The listing builds one solid part. Answer for the finished solid, in the listing's coordinates (mm). A direction names the side the tool comes from. Round coordinates to 2 decimals unless told otherwise and drop trailing zeros. Order: outer loops, then holes, each group sorted by start corner. A loop starts at its lowest first (then second) coordinate and runs counter-clockwise, first axis right, second up. Notation, with made-up numbers: M 84.25,57.25 L 111.25,57.25 A18 ccw 111.25,76.25 Z; hole C 3,19.25 d3. An arc over 180 degrees is marked long. Write item = value, one per line. Start each with the question number.
(1) A cutting plane is placed at B-B, the plane z = 83. Determine the outline of the cut face in (x, y), and give its area (3 significant figures).
(2) Which of the six approach directions +Z, -Z, +X, -X, +Y, -Y give full straight-line access (tool end or side, diameter ignored) to faces 1 (the face through (0, -17, 72.215)), 2 (the face through (0, 0, 5)), 3 (the face through (0, -3, 25)), 4 (the face through (-0.434, -36.93, 68.934))?
(3) A cutting plane is placed at D-D, the plane z = 98. Determine the outline of the cut face in (x, y) (1 decimal).
(4) A cutting plane is placed at A-A, the plane x = 5.75. Determine the outline of the cut face in (y, z), and give its area (3 significant figures).
(5) Straight lines are drawn through the part: probe 1 along Z at (x, y) = (-2.5, -22); probe 2 along Y at (x, z) = (-0.75, 79.5); probe 3 along Z at (x, y) = (-0.25, -35). For each, find the intervals that lie inside material, in ascending order. Write a range as from..to.
(6) A cutting plane is placed at C-C, the plane y = -16.5. Determine the outline of the cut face in (x, z).
(7) Each of these flat-tipped pins is pushed along its axis until it touches: pin 1 (12.5 mm diameter, centred on x = 1.5, z = 61, fed in from +Y); pin 2 (3 mm diameter, centred on x = 3.5, z = 69, fed in from -Y); pin 3 (6 mm diameter, centred on x = 8.5, y = -30.5, fed in from -Z). Where does it stop, or does it pass through?
Autodesk Inventor part; units mm, degrees
ref_plane "YZ Plane" through (0, 0, 0) normal (1, 0, 0) x (0, 1, 0)
ref_plane "XZ Plane" through (0, 0, 0) normal (0, 1, 0) x (-1, 0, 0)
ref_plane "XY Plane" through (0, 0, 0) normal (0, 0, 1) x (1, 0, 0)
sketch "Sketch1" plane through (0, 0, 0) normal (0, 0, 1) x (1, 0, 0)
  circle A0 centre (0, 0) radius 3
  dimension "d0" = 6
extrude "Extrusion1" add sketch "Sketch1" along normal blind 50
sketch "Sketch2" plane through (0, 0, 0) normal (0, 1, 0) x (-1, 0, 0)
  line L0 (-12.5, 75) -> (-12.5, 50)
  line L1 (-12.5, 50) -> (12.5, 50)
  line L2 (12.5, 50) -> (12.5, 75)
  line L3 (12.5, 75) -> (-12.5, 75)
  line L4 (-12.5, 75) -> (12.5, 50) construction
  line L5 (-12.5, 50) -> (12.5, 75) construction
  line L6 (3, 50) -> (-3, 50)
  line L7 (3, 50) -> (-3, 50)
  line L8 (3, 0) -> (-3, 0)
  line L9 (3, 0) -> (-3, 0)
  line L10 (-3, 0) -> (3, 50)
  line L11 (3, 0) -> (-3, 50)
  line L12 (12.5, 75) -> (3, 84.5)
  line L13 (3, 84.5) -> (3, 84.5)
  line L14 (3, 84.5) -> (-3, 84.5)
  line L15 (-3, 84.5) -> (-3, 84.5)
  line L16 (-3, 84.5) -> (-12.5, 75)
  line L17 (0.25, 84.5) -> (0, 114.5)
  line L18 (0, 114.5) -> (-0.25, 84.5)
  line L19 (0, 114.5) -> (0, 84.5)
  point P0 (0, 0)
  point P1 (0, 62.5)
  point P2 (0, 50)
  point P3 (0, 25)
  point P4 (0, 62.5)
  dimension "d3" = 25
  dimension "d4" = 25
  dimension "d5" = 6
  dimension "d6" = 0
  dimension "d11" = 30
  dimension "d14" = 0.5
  dimension "d15" = 0.25
extrude "Extrusion2" add sketch "Sketch2" along normal mid plane 4 contours L3 L2 L1 L0 | L16 L14 L12 L3
sketch "Sketch3" plane through (0, -2, 0) normal (0, -1, 0) x (1, 0, 0)
  line L0 (-10, 72.2148) -> (-10, 62.2148)
  line L1 (-10, 62.2148) -> (10, 62.2148)
  line L2 (10, 62.2148) -> (10, 72.2148)
  line L3 (10, 72.2148) -> (-10, 72.2148)
  line L4 (-10, 72.2148) -> (10, 62.2148) construction
  line L5 (-10, 62.2148) -> (10, 72.2148) construction
  point P0 (0, 0)
  point P1 (0, 67.2148)
  dimension "d18" = 10
  dimension "d24" = 20
extrude "Extrusion3" add sketch "Sketch3" along normal blind 30
revolve "Revolution1" add sketch "Sketch2" angle 360 about axis through (0, 0, 114.5) along (0, 0, -1) contours L14 L19 L17
sketch "Sketch5" plane through (0, 0, 0) normal (0, 0, -1) x (-1, 0, 0)
  arc A0 (-2.2361, 2) -> (-2.2361, -2) centre (0, 0) ccw
  line L0 (-3, 0) -> (3.9396, 0)
  line L1 (3.9396, 0) -> (3.9396, 5.4672)
  line L2 (3.9396, 5.4672) -> (-3, 5.4672)
  line L3 (-3, 5.4672) -> (-3, 0)
extrude "Extrusion4" cut sketch "Sketch5" against normal blind 10
sketch "Sketch6" plane through (0, -32, 0) normal (0, -1, 0) x (1, 0, 0)
  circle A0 centre (0, 66.9819) radius 2
  point P0 (0, 0)
  dimension "d25" = 4
extrude "Extrusion5" add sketch "Sketch6" along normal blind 10
equation "\"d15\" = 0.5 * d14"
properties part number "electrode"
Reported:
q1.outline = M -4.5,-2 L 4.5,-2 L 4.5,2 L -4.5,2 Z
q1.area = 36.0 mm²
q2.face_1 = +Z, +X, -X, -Y
q2.face_2 = -Z, +X, -X, +Y
q2.face_3 = -Z
q2.face_4 = -Y
q3.outline = C 0,0 d0.3
q4.outline = M -32,62.21 L -2,62.21 L -2,50 L 2,50 L 2,81.75 L -2,81.75 L -2,72.21 L -32,72.21 Z
q4.area = 427 mm²
q5.probe_1 = 62.21..72.21
q5.probe_2 = -2..2
q5.probe_3 = 65..68.97
q6.outline = M -10,62.21 L 10,62.21 L 10,72.21 L -10,72.21 Z
q7.pin_1 = 2
q7.pin_2 = -32
q7.pin_3 = 62.21
